CAD build for the part. Positions are in the model's coordinates, mm. A direction names the side the tool comes from. Round coordinates to 2 decimals unless told otherwise and drop trailing zeros. Write each loop counter-clockwise with the first axis right and the second up, starting at its lowest first coordinate (ties: lowest second). Pieces come first, ordered by that corner, then holes. Notation, with made-up numbers: (-0.75, -24.5) -> (9.25, -24.5) arc R29 ccw to (9.25, 1.5) -> close; hole circle Ø8 at (62, -23.75). An arc over 180 degrees is marked (long way). Answer in a Markdown table with one row per item. Add a question column.
```python
from build123d import *

# Parameters (mm, degrees)
F1_DEPTH = 6
F3_DEPTH = 5.4
F4_SIZE  = 0.5


with BuildPart() as f1:
    # F0 (on Top) → F1 (new body)
    with BuildSketch(Plane.XY):
        with BuildLine():
            Line((13.25, 18.9), (-13.25, 18.9))
            ThreePointArc((-13.25, 18.9), (-26.6143181644, 13.3643181644), (-32.15, 0))
            ThreePointArc((-32.15, 0), (-26.6143181644, -13.3643181644), (-13.25, -18.9))
            Line((-13.25, -18.9), (13.25, -18.9))
            ThreePointArc((13.25, -18.9), (26.6143181644, -13.3643181644), (32.15, 0))
            ThreePointArc((32.15, 0), (26.6143181644, 13.3643181644), (13.25, 18.9))
        make_face()
    extrude(amount=F1_DEPTH)

    # F2 (on face) → F3 (cut)
    with BuildSketch(Plane.XY.offset(6)):
        with BuildLine():
            Line((13.25, 18.1), (-13.25, 18.1))
            ThreePointArc((-13.25, 18.1), (-31.35, 0), (-13.25, -18.1))
            Line((-13.25, -18.1), (13.25, -18.1))
            ThreePointArc((13.25, -18.1), (31.35, 0), (13.25, 18.1))
        make_face()
    extrude(amount=-F3_DEPTH, mode=Mode.SUBTRACT)

    # F4
    f4_edges = [f1.edges().sort_by_distance(p)[0] for p in [
        (-32.15, 0, 6),
        (32.15, 0, 6),
        (0, 18.9, 6),
        (0, -18.9, 6),
    ]]
    chamfer(f4_edges, length=F4_SIZE)


solid = f1.part
```
Item 1: Saw through at B-B on x = 5. Give the cut face in (y, z), then the cut area to 3 significant figures.
Item 2: Pin check, flat tips, straight feed: pin 1 (8 mm diameter, centred on x = -13.5, y = -2.5, fed in from +Z); pin 2 (2 mm diameter, centred on x = -23.5, z = 5, fed in from -Y); pin 3 (1.5 mm diameter, centred on x = 23, z = 3, fed in from +Y). Stop position of each tip, or through.
Item 3: Tool access for faces 1 (the flat face through (0, -18.1, 3)), 2 (the flat face through (0, 18.9, 3)): list every direction of +Z, -Z, +X, -X, +Y, -Y with a clear straight run to the whole face (end or side of a thin tool).
Item 4: Drill centre lines: probe 1 along Y at (x, z) = (-8, 1); probe 2 along Z at (x, y) = (10.5, 11.5); probe 3 along X at (y, z) = (-2.5, 4.75). Where is each one in solid material? Low to high.
Item 5: Two-plate mould, pull along X, no slides. Class faces 3 (the flat face through (0, 0, 0)), 4 (the cylindrical face through (-31.346, 0.398, 3.338)): +X half, -X half, draft (parallel to the pull), parting line (faces both ways), or undercut.
Item 6: Saw through at A-A on z = 2.25. Give the cut face in (x, y).
Recorded:
| question | item | result |
|---|---|---|
| 1 | outline | (-18.9, 0) -> (18.9, 0) -> (18.9, 5.5) -> (18.4, 6) -> (18.1, 6) -> (18.1, 0.6) -> (-18.1, 0.6) -> (-18.1, 6) -> (-18.4, 6) -> (-18.9, 5.5) -> close |
| 1 | area | 31.1 mm2 |
| 2 | pin 1 | z = 0.6 |
| 2 | pin 2 | y = -16.48 |
| 2 | pin 3 | y = 16.62 |
| 3 | face 1 | +Z |
| 3 | face 2 | +Z, -Z, +X, -X, +Y |
| 4 | probe 1 | -18.9 to -18.1, 18.1 to 18.9 |
| 4 | probe 2 | 0 to 0.6 |
| 4 | probe 3 | -31.98 to -31.18, 31.18 to 31.98 |
| 5 | face 3 | draft |
| 5 | face 4 | undercut |
| 6 | outline | (-13.25, -18.9) -> (13.25, -18.9) arc R18.9 ccw to (13.25, 18.9) -> (-13.25, 18.9) arc R18.9 ccw to start; hole (-13.25, -18.1) -> (13.25, -18.1) arc R18.1 ccw to (13.25, 18.1) -> (-13.25, 18.1) arc R18.1 ccw to start |
